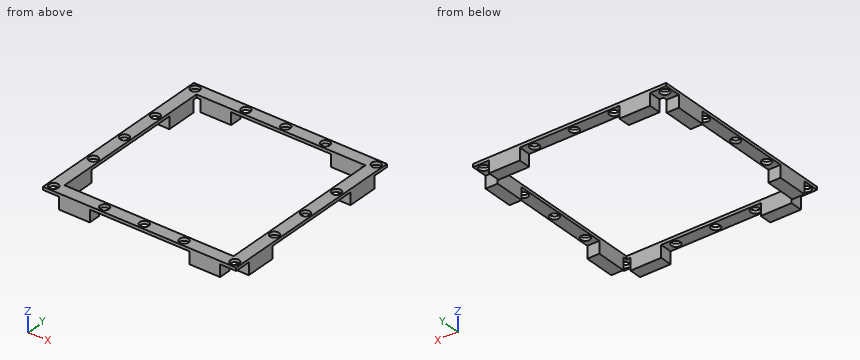
Autodesk Inventor part; units mm, degrees
ref_plane "YZ Plane" through (0, 0, 0) normal (1, 0, 0) x (0, 1, 0)
ref_plane "XZ Plane" through (0, 0, 0) normal (0, 1, 0) x (-1, 0, 0)
ref_plane "XY Plane" through (0, 0, 0) normal (0, 0, 1) x (1, 0, 0)
sketch "Sketch1" plane through (0, 0, 0) normal (0, 0, 1) x (1, 0, 0)
  line L0 (-48, 48) -> (48, 48)
  line L1 (48, 48) -> (48, -48)
  line L2 (48, -48) -> (-48, -48)
  line L3 (-48, -48) -> (-48, 48)
  line L4 (42, 42) -> (-42, 42)
  line L5 (-42, 42) -> (-42, -42)
  line L6 (-42, -42) -> (42, -42)
  line L7 (42, -42) -> (42, 42)
  line L8 (0, 152.7233) -> (0, -72.1628) construction
  line L9 (-77.8847, 0) -> (88.8171, 0) construction
  line L10 (-48, 45) -> (48, 45) construction
  circle A0 centre (0, 45) radius 2.25
  circle A1 centre (-19.75, 45) radius 2.25
  circle A2 centre (19.75, 45) radius 2.25
  line L11 (-45, 48) -> (-45, -48) construction
  circle A3 centre (-45, 45) radius 2.25
  circle A4 centre (-45, 0) radius 2.25
  line L12 (-48, -45) -> (48, -45) construction
  circle A5 centre (-45, -45) radius 2.25
  circle A6 centre (-45, 19.75) radius 2.25
  circle A7 centre (-45, -19.75) radius 2.25
  point P0 (0, 0)
  point P1 (0, 48)
  point P2 (48, 0)
  dimension "d0" = 96
  dimension "d1" = 96
  dimension "d2" = 6
  dimension "d5" = 3
  dimension "d6" = 4.5
  dimension "d7" = 4.5
  dimension "d8" = 4.5
  dimension "d9" = 22
  dimension "d10" = 22
  dimension "d11" = 3
  dimension "d12" = 4.5
  dimension "d13" = 4.5
  dimension "d14" = 3
  dimension "d15" = 4.5
  dimension "d31" = 4.5
  dimension "d32" = 4.5
  dimension "d33" = 22
  dimension "d34" = 22
extrude "Extrusion1" add sketch "Sketch1" along normal blind 1.5 contours L0 L1 L2 L3 | A0 | A1 | A2 | A3 | A4 | A5 | A6 | A7
extrude "Extrusion2" cut sketch "Sketch1" along normal blind 10 contours A0 | A1 | A2
mirror "Mirror1" about plane through (0, 0, 0) normal (0, 1, 0) of "Extrusion2"
extrude "Extrusion3" cut sketch "Sketch1" along normal blind 10 contours A3 | A4 | A5 | A6 | A7
mirror "Mirror2" about plane through (0, 0, 0) normal (1, 0, 0) of "Extrusion3"
sketch "Sketch2" plane through (0, 0, 0) normal (0, 0, -1) x (-1, 0, 0)
  circle A0 centre (-45, 19.75) radius 2.25
  circle A1 centre (-45, 0) radius 2.25
  circle A2 centre (-45, 45) radius 2.25
  circle A3 centre (0, 45) radius 2.25
  circle A4 centre (-19.75, 45) radius 2.25
  line L0 (48, 48) -> (-48, 48)
  line L1 (-48, 48) -> (-48, -48)
  line L2 (-42, -42) -> (-42, 42)
  line L3 (-42, 42) -> (42, 42)
  line L4 (-48, 40) -> (-42, 40)
  line L5 (-42, 40) -> (-42, 24.75)
  line L6 (-42, 24.75) -> (-48, 24.75)
  line L7 (-48, 24.75) -> (-48, 40)
  line L8 (-48, 14.75) -> (-42, 14.75)
  line L9 (-42, 14.75) -> (-42, 5)
  line L10 (-42, 5) -> (-48, 5)
  line L11 (-48, 5) -> (-48, 14.75)
  line L12 (-40, 48) -> (-24.75, 48)
  line L13 (-24.75, 48) -> (-24.75, 42)
  line L14 (-24.75, 42) -> (-40, 42)
  line L15 (-40, 42) -> (-40, 48)
  line L16 (-14.75, 48) -> (-5, 48)
  line L17 (-5, 48) -> (-5, 42)
  line L18 (-5, 42) -> (-14.75, 42)
  line L19 (-14.75, 42) -> (-14.75, 48)
  dimension "d35" = 5
  dimension "d36" = 5
  dimension "d37" = 5
  dimension "d38" = 5
  dimension "d39" = 5
  dimension "d40" = 5
  dimension "d41" = 5
  dimension "d42" = 5
extrude "Extrusion4" add sketch "Sketch2" along normal blind 6 contours L13 L3 L15 L0 | L4 L2 L6 L1
mirror "Mirror3" about plane through (0, 0, 0) normal (1, 0, 0) of "Extrusion4"
mirror "Mirror4" about plane through (0, 0, 0) normal (0, 1, 0) of "Extrusion4", "Mirror3"
properties part number "Base" material "ABS Plastic"
Geometry: final body of the model. Coordinates: model frame, mm. Round coordinates to 2 decimals unless told otherwise and drop trailing zeros. Write each loop counter-clockwise with the first axis right and the second up, starting at its lowest first coordinate (ties: lowest second). Pieces come first, ordered by that corner, then holes. Notation, with made-up numbers: M 8.25,50.5 L 45.25,50.5 A29 cw 45.25,73.5 Z; hole C 7,61.5 d6. An arc over 180 degrees is marked long. Answer in a Markdown table with one row per item. Add a question column.
(1) Cut plane B-B, the plane x = 19.75. Return the cut outline in (y, z).
(2) Cut plane C-C, the plane y = 10.5. Return the cut outline in (x, z), then the cut area to 3 significant figures.
(3) Ray query, L1, parallel to Y at x = 45, z = 0.55; L2, parallel to Y at x = 19.75, z = 0.9; L3, parallel to X at y = -30.5, z = 0. Return the intervals inside material, ascending.
(4) Contact query for flat-ended pins moving along their axis: pin 1 (6.5 mm diameter, centred on x = 43.5, y = 45.5, fed in from -Z); pin 2 (1.8 mm diameter, centred on y = -46.5, z = -2.5, fed in from -X); pin 3 (1.8 mm diameter, centred on x = 44, z = -3.5, fed in from -Y). Output: stop coordinate, or through.
(5) Cut plane A-A, the plane y = 45. Give the number of separate pieces and of enclosed holes in the cut face, then the cut area to 3 significant figures.
Established:
| question | item | result |
|---|---|---|
| 1 | outline | M -48,0 L -47.25,0 L -47.25,1.5 L -48,1.5 Z; M -42.75,0 L -42,0 L -42,1.5 L -42.75,1.5 Z; M 42,0 L 42.75,0 L 42.75,1.5 L 42,1.5 Z; M 47.25,0 L 48,0 L 48,1.5 L 47.25,1.5 Z |
| 2 | outline | M -48,0 L -42,0 L -42,1.5 L -48,1.5 Z; M 42,0 L 48,0 L 48,1.5 L 42,1.5 Z |
| 2 | area | 18.0 mm² |
| 3 | L1 | -48 to -47.25, -42.75 to -22, -17.5 to -2.25, 2.25 to 17.5, 22 to 42.75, 47.25 to 48 |
| 3 | L2 | -48 to -47.25, -42.75 to -42, 42 to 42.75, 47.25 to 48 |
| 3 | L3 | -48 to -42, 42 to 48 |
| 4 | pin 1 | z = 0 |
| 4 | pin 2 | x = -40 |
| 4 | pin 3 | y = -40 |
| 5 | separate pieces | 6 |
| 5 | enclosed holes | 0 |
| 5 | area | 293 mm² |
